Read the model definition and answer for the solid it produces. Units are mm, in the model's axes. Face numbers are marked on the shaded views. A direction names the side the tool comes from. Round coordinates to 2 decimals unless told otherwise and drop trailing zeros. Order: outer loops, then holes, each group sorted by start corner. A loop starts at its lowest first (then second) coordinate and runs counter-clockwise, first axis right, second up. Notation, with made-up numbers: M -29.5,32.25 L 7.5,32.25 A14 ccw 7.5,53.25 Z; hole C -38,-19 d4. An arc over 180 degrees is marked long. Answer as CSV lines item,"result".
```python
from build123d import *

# Parameters (mm, degrees)
SKETCH_4_W          = 40
SKETCH_4_H          = 65
EXTRUDE_1_DEPTH     = 3
SKETCH_5_R          = 5.05
CUT_EXTRUDE_1_DEPTH = 2
SKETCH_6_R          = 1.5
SKETCH_6_R_2        = 1
CUT_EXTRUDE_2_DEPTH = 1
SKETCH_6_2_R        = 1
CUT_EXTRUDE_3_DEPTH = 39.278584091
SKETCH_7_W          = 7
SKETCH_7_H          = 12
EXTRUDE_2_DEPTH     = 5
SKETCH_8_R          = 5.5
CUT_EXTRUDE_4_DEPTH = 5.5
CUT_EXTRUDE_START   = -23.5
SKETCH_8_2_R        = 5.5
CUT_EXTRUDE_5_DEPTH = 5.5


with BuildPart() as part:
    # 草图4 → 凸台-拉伸1 (new body)
    with BuildSketch(Plane(origin=(0, 0, 0), x_dir=(1, 0, 0), z_dir=(0, 1, 0))):
        Rectangle(SKETCH_4_W, SKETCH_4_H)
    extrude(amount=EXTRUDE_1_DEPTH)

    # 草图5 → 切除-拉伸1 (cut)
    with BuildSketch(Plane.XZ):
        with Locations(Location((-12, 22.5, 0), (0, 0, 270))):
            Circle(SKETCH_5_R)
        with Locations(Location((12, 22.5, 0), (0, 0, 270))):
            Circle(SKETCH_5_R)
        with Locations(Location((12, -22.5, 0), (0, 0, 270))):
            Circle(SKETCH_5_R)
        with Locations(Location((-12, -22.5, 0), (0, 0, 270))):
            Circle(SKETCH_5_R)
    extrude(amount=-CUT_EXTRUDE_1_DEPTH, mode=Mode.SUBTRACT)

    # 草图6 → 切除-拉伸2 (cut)
    # profile 1 of 4: a face of its own
    with BuildSketch(Plane(origin=(0, 3, 0), x_dir=(1, 0, 0), z_dir=(0, 1, 0))):
        with Locations(Location((-18.1, 30, 0), (0, 0, 270))):
            Circle(SKETCH_6_R)
        with Locations(Location((-18.1, 30, 0), (0, 0, 270))):
            Circle(SKETCH_6_R_2, mode=Mode.SUBTRACT)
    # profile 2 of 4: a face of its own
    with BuildSketch(Plane(origin=(0, 3, 0), x_dir=(1, 0, 0), z_dir=(0, 1, 0))):
        with Locations(Location((18.1, 30, 0), (0, 0, 270))):
            Circle(SKETCH_6_R)
        with Locations(Location((18.1, 30, 0), (0, 0, 270))):
            Circle(SKETCH_6_R_2, mode=Mode.SUBTRACT)
    # profile 3 of 4: a face of its own
    with BuildSketch(Plane(origin=(0, 3, 0), x_dir=(1, 0, 0), z_dir=(0, 1, 0))):
        with Locations(Location((-18.1, -30, 0), (0, 0, 270))):
            Circle(SKETCH_6_R)
        with Locations(Location((-18.1, -30, 0), (0, 0, 270))):
            Circle(SKETCH_6_R_2, mode=Mode.SUBTRACT)
    # profile 4 of 4: a face of its own
    with BuildSketch(Plane(origin=(0, 3, 0), x_dir=(1, 0, 0), z_dir=(0, 1, 0))):
        with Locations(Location((18.1, -30, 0), (0, 0, 270))):
            Circle(SKETCH_6_R)
        with Locations(Location((18.1, -30, 0), (0, 0, 270))):
            Circle(SKETCH_6_R_2, mode=Mode.SUBTRACT)
    extrude(amount=-CUT_EXTRUDE_2_DEPTH, mode=Mode.SUBTRACT)

    # 草图6<2> → 切除-拉伸3 (cut, through all)
    with BuildSketch(Plane(origin=(0, 3, 0), x_dir=(1, 0, 0), z_dir=(0, 1, 0))):
        with Locations(Location((-18.1, -30, 0), (0, 0, 270))):
            Circle(SKETCH_6_2_R)
        with Locations(Location((18.1, -30, 0), (0, 0, 270))):
            Circle(SKETCH_6_2_R)
        with Locations(Location((18.1, 30, 0), (0, 0, 270))):
            Circle(SKETCH_6_2_R)
        with Locations(Location((-18.1, 30, 0), (0, 0, 270))):
            Circle(SKETCH_6_2_R)
    extrude(amount=-CUT_EXTRUDE_3_DEPTH, mode=Mode.SUBTRACT)

    # 草图7 → 凸台-拉伸2 (add)
    with BuildSketch(Plane(origin=(0, 3, 0), x_dir=(1, 0, 0), z_dir=(0, 1, 0))):
        with Locations((-11, 16.5)):
            Rectangle(SKETCH_7_W, SKETCH_7_H)
        with Locations((11, 16.5)):
            Rectangle(SKETCH_7_W, SKETCH_7_H)
        with Locations((11, -17.5)):
            Rectangle(SKETCH_7_W, SKETCH_7_H)
        with Locations((-11, -17.5)):
            Rectangle(SKETCH_7_W, SKETCH_7_H)
    extrude(amount=EXTRUDE_2_DEPTH)

    # 草图8 → 切除-拉伸4 (cut)
    with BuildSketch(Plane.ZY.offset(14.5)):
        with Locations((-16.5, 8)):
            Circle(SKETCH_8_R)
        with Locations((17.5, 8)):
            Circle(SKETCH_8_R)
    extrude(amount=-CUT_EXTRUDE_4_DEPTH, mode=Mode.SUBTRACT)

    # 草图8<2> → 切除-拉伸5 (cut)
    with BuildSketch(Plane.ZY.offset(14.5).offset(CUT_EXTRUDE_START)):
        with Locations((-16.5, 8)):
            Circle(SKETCH_8_2_R)
        with Locations((17.5, 8)):
            Circle(SKETCH_8_2_R)
    extrude(amount=-CUT_EXTRUDE_5_DEPTH, mode=Mode.SUBTRACT)


solid = part.part
```
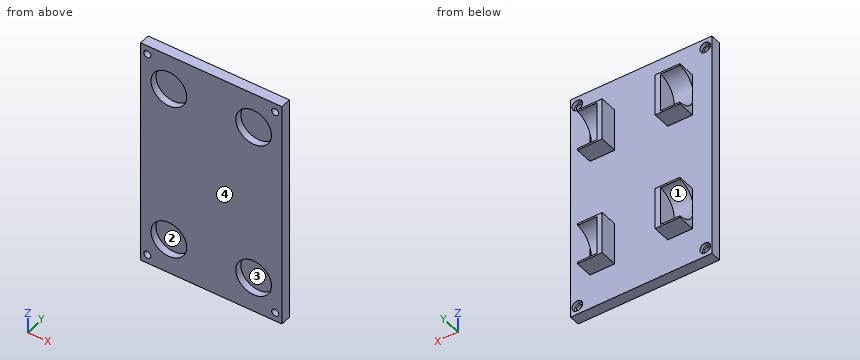
Item 1: Find the intervals of material crossed by probe 1 along X at (y, z) = (2.7, -30); probe 2 along X at (y, z) = (1.2, 22.5); probe 3 along X at (y, z) = (5, 14), in increasing order. Write a range as [from, to].
Ans:
probe 1,"[-20, -19.6], [-16.6, 16.6], [19.6, 20]"
probe 2,"[-20, -17.05], [-6.95, 6.95], [17.05, 20]"
probe 3,"[-9, -7.5], [7.5, 9]"
Item 2: Determine the mould class of the marked faces 3 and 4 for opening direction X: +X half, -X half, draft (parallel to the pull), parting line (faces both ways), or undercut.
Ans:
face 3,"undercut"
face 4,"draft"
Item 3: A cutting plane is placed at A-A, the plane x = 18.1. Determine the outline of the cut face in (y, z), and give its area (3 significant figures).
Ans:
outline,"M 0,-32.5 L 3,-32.5 L 3,-31.5 L 2,-31.5 L 2,-31 L 0,-31 Z; M 0,-29 L 2,-29 L 2,-28.5 L 3,-28.5 L 3,28.5 L 2,28.5 L 2,29 L 0,29 Z; M 0,31 L 2,31 L 2,31.5 L 3,31.5 L 3,32.5 L 0,32.5 Z"
area,"181 mm2"
Item 4: A cutting plane is placed at D-D, the plane z = 30. Determine the outline of the cut face in (x, y), and give its area (3 significant figures).
Ans:
outline,"M -20,0 L -19.1,0 L -19.1,2 L -19.6,2 L -19.6,3 L -20,3 Z; M -17.1,0 L 17.1,0 L 17.1,2 L 16.6,2 L 16.6,3 L -16.6,3 L -16.6,2 L -17.1,2 Z; M 19.1,0 L 20,0 L 20,3 L 19.6,3 L 19.6,2 L 19.1,2 Z"
area,"106 mm2"
Item 5: A tool of negligible diameter and unlimited length cuts with its end or side. For the marked faces 1 and 2, from which of +Z, -Z, +X, -X, +Y, -Y can it reach the whole face along a straight path? Write none if from no direction.
Ans:
face 1,"+Y"
face 2,"-Y"
Item 6: Flat-ended cylindrical pins translate along their axes: pin 1 (3 mm diameter, centred on y = 6, z = 21.5, fed in from +X); pin 2 (2.5 mm diameter, centred on y = 5, z = 20, fed in from +X); pin 3 (1.5 mm diameter, centred on y = 5, z = 18.5, fed in from -X). Find the tip coordinate at first contact, or state that the pin passes through.
Ans:
pin 1,"x = 14.5"
pin 2,"x = 9"
pin 3,"x = -9"
Item 7: A cutting plane is placed at B-B, the plane z = -16.5. Determine the outline of the cut face in (x, y), and give its area (4 significant figures).
Ans:
outline,"M -20,0 L 20,0 L 20,3 L 14.5,3 L 14.5,2.5 L 9,2.5 L 9,8 L 7.5,8 L 7.5,3 L -7.5,3 L -7.5,8 L -9,8 L -9,2.5 L -14.5,2.5 L -14.5,3 L -20,3 Z"
area,"129.5 mm2"
Item 8: A cutting plane is placed at C-C, the plane y = 0.75. Give the number of separate pieces and of enclosed holes in the cut face, and give its area (3 significant figures).
Ans:
separate pieces,"1"
enclosed holes,"8"
area,"2,270 mm2"
